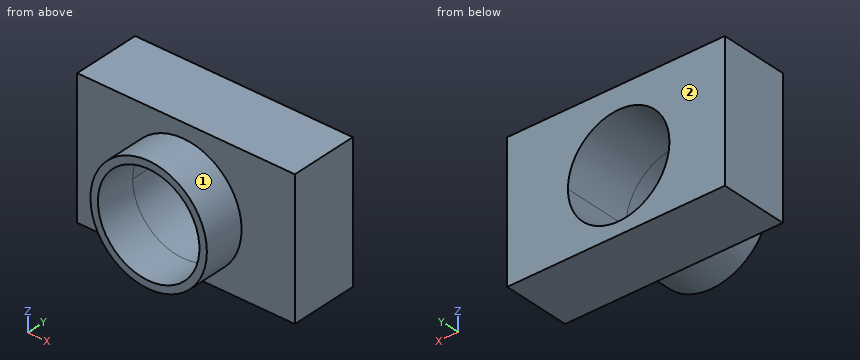
from build123d import *

# Parameters (mm, degrees)
F0_W     = 80
F0_H     = 50
F1_DEPTH = 25
F2_R     = 18.6615462825
F3_DEPTH = 45.6
F4_R     = 21.4002075556
F4_R_2   = 18.6615462825
F5_DEPTH = 40


with BuildPart() as f1:
    # F0 (on Front) → F1 (new body)
    with BuildSketch(Plane.XZ):
        with Locations((0.9671058506, -12.7448502543)):
            Rectangle(F0_W, F0_H)
    extrude(amount=F1_DEPTH)

    # F2 (on Front) → F3 (cut, symmetric)
    with BuildSketch(Plane.XZ):
        with Locations((0, -14.5065793768)):
            Circle(F2_R)
    extrude(amount=F3_DEPTH, both=True, mode=Mode.SUBTRACT)

    # F4 (on face) → F5 (join)
    with BuildSketch(Plane(origin=(0, 0, 0), x_dir=(-1, 0, 0), z_dir=(0, 1, 0))):
        with Locations((0, -14.5065793768)):
            Circle(F4_R)
        with Locations((0, -14.5065793768)):
            Circle(F4_R_2, mode=Mode.SUBTRACT)
    extrude(amount=-F5_DEPTH)


solid = f1.part
Design review of the part built by this model. Coordinates are the model's own, in mm. Face numbers are marked on the shaded views. A direction names the side the tool comes from. Give positions to 0.01 mm unless a question says otherwise; leave off trailing zeros. Loops run counter-clockwise (first coordinate to the right, second up) from the corner with the lowest first, then second, coordinate; pieces in that order, holes last. Notation, with made-up numbers: (19, 12) -> (45, 12) arc R19 ccw to (45, 48) -> close; hole circle Ø4 at (-24.75, 66). An arc over 180 degrees is marked (long way). One line per question, with ' | ' between items. Start each with the question number.
(1) We need section A-A (x = 0). State the section outline as (y, z) points.
(2) We need section D-D (x = 27.5). State the section outline as (y, z) points.
(3) For line 1 (Z direction, x = 0, y = -32.5); line 2 (Y direction, x = 33, z = -24); line 3 (Z direction, x = -12.5, y = -5), list the stretches that pass through material, from the lowest coordinate up.
(4) We need section B-B (z = -15.5). State the section outline as (x, y) points, and give its area (3 significant figures).
(5) We need section C-C (y = -7.5). State the section outline as (x, z) points.
(6) Insertion check: P1, Ø3, axis at x = 23.5, z = -14, coming from the -Y side; P2, Ø3, axis at x = -13, y = -27.5, coming from the -Z side. Each pin has a flat end and moves straight along its axis. Give the tip position at first contact, or say it passes through.
(7) For the marked faces 1 and 2, list the 3-axis set-ups (+Z, -Z, +X, -X, +Y, -Y) from which the entire face can be reached by the end or side of a thin tool; tool diameter is ignored.
The answers:
1) outline: (-40, -35.91) -> (-25, -35.91) -> (-25, -37.74) -> (0, -37.74) -> (0, -33.17) -> (-40, -33.17) -> close; (-40, 4.15) -> (0, 4.15) -> (0, 12.26) -> (-25, 12.26) -> (-25, 6.89) -> (-40, 6.89) -> close
2) outline: (-25, -37.74) -> (0, -37.74) -> (0, 12.26) -> (-25, 12.26) -> close
3) line 1: z = -35.91 to -33.17, 4.15 to 6.89 | line 2: y = -25 to 0 | line 3: z = -37.74 to -28.36, -0.65 to 12.26
4) outline: (-39.03, -25) -> (-21.38, -25) -> (-21.38, -40) -> (-18.64, -40) -> (-18.64, 0) -> (-39.03, 0) -> close; (18.64, -40) -> (21.38, -40) -> (21.38, -25) -> (40.97, -25) -> (40.97, 0) -> (18.64, 0) -> close | area: 1,150 mm^2
5) outline: (-39.03, -37.74) -> (40.97, -37.74) -> (40.97, 12.26) -> (-39.03, 12.26) -> close; hole circle Ø37.32 at (0, -14.51)
6) P1: stops at y = -25 | P2: stops at z = -32.55
7) face 1: -Y | face 2: +Z, -Z, +X, -X, +Y
